For this review, take the finished solid that the model builds, in its own axes (mm). Face numbers are marked on the shaded views. Round coordinates to 2 decimals unless told otherwise and drop trailing zeros. Order: outer loops, then holes, each group sorted by start corner. A loop starts at its lowest first (then second) coordinate and runs counter-clockwise, first axis right, second up. Notation, with made-up numbers: (29.25, 32.25) -> (46.25, 32.25) arc R12 ccw to (46.25, 54.25) -> close; hole circle Ø6 at (-39, -12). An arc over 180 degrees is marked (long way). Answer in a Markdown table with one row per item.
```python
from build123d import *

# Parameters (mm, degrees)
SKETCH1_W           = 22
SKETCH1_H           = 6.5
SKETCH1_R           = 1.5
BOSS_EXTRUDE1_DEPTH = 2.5
FILLET4_R           = 2


with BuildPart() as part:
    # Sketch1 → Boss-Extrude1 (new body)
    with BuildSketch(Plane.XY):
        Rectangle(SKETCH1_W, SKETCH1_H)
        with Locations((-8.75, 0)):
            Circle(SKETCH1_R, mode=Mode.SUBTRACT)
        with Locations(Location((8.75, 0, 0), (0, 0, 180))):
            Circle(SKETCH1_R, mode=Mode.SUBTRACT)
    extrude(amount=BOSS_EXTRUDE1_DEPTH)

    # Fillet4
    fillet4_edges = [part.edges().sort_by_distance(p)[0] for p in [
        (11, -3.25, 1.25),
        (-11, -3.25, 1.25),
        (-11, 3.25, 1.25),
        (11, 3.25, 1.25),
    ]]
    fillet(fillet4_edges, radius=FILLET4_R)


solid = part.part
```
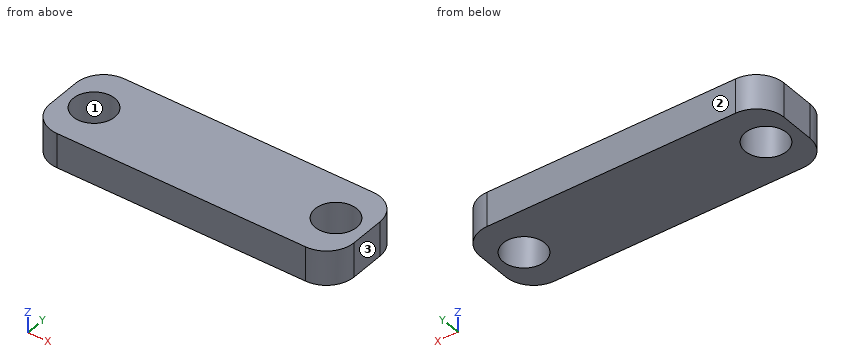
Q1. Take a section at D-D, the plane y = 0.25. Write out the cut boundary in (x, z).
Answer key:
| item | result |
|---|---|
| outline | (-11, 0) -> (-10.23, 0) -> (-10.23, 2.5) -> (-11, 2.5) -> close; (-7.27, 0) -> (7.27, 0) -> (7.27, 2.5) -> (-7.27, 2.5) -> close; (10.23, 0) -> (11, 0) -> (11, 2.5) -> (10.23, 2.5) -> close |
Q2. Take a section at A-A, the plane z = 0.6. Write out the cut boundary in (x, y), then the cut area to 3 significant figures.
Answer key:
| item | result |
|---|---|
| outline | (-11, -1.25) arc R2 ccw to (-9, -3.25) -> (9, -3.25) arc R2 ccw to (11, -1.25) -> (11, 1.25) arc R2 ccw to (9, 3.25) -> (-9, 3.25) arc R2 ccw to (-11, 1.25) -> close; hole circle Ø3 at (-8.75, 0); hole circle Ø3 at (8.75, 0) |
| area | 125 mm^2 |
Q3. The part is to be moulded in two halves that separate along X. For the marked faces 1, 2 and 3, say which applies: +X half, -X half, draft (parallel to the pull), parting line (faces both ways), or undercut.
Answer key:
| item | result |
|---|---|
| face 1 | undercut |
| face 2 | draft |
| face 3 | +X half |
Q4. Take a section at B-B, the plane x = 8.75. Write out the cut boundary in (y, z), then the cut area to 3 significant figures.
Answer key:
| item | result |
|---|---|
| outline | (-3.25, 0) -> (-1.5, 0) -> (-1.5, 2.5) -> (-3.25, 2.5) -> close; (1.5, 0) -> (3.25, 0) -> (3.25, 2.5) -> (1.5, 2.5) -> close |
| area | 8.75 mm^2 |
Q5. Take a section at C-C, the plane y = -0.75. Write out the cut boundary in (x, z), then the cut area to 3 significant figures.
Answer key:
| item | result |
|---|---|
| outline | (-11, 0) -> (-10.05, 0) -> (-10.05, 2.5) -> (-11, 2.5) -> close; (-7.45, 0) -> (7.45, 0) -> (7.45, 2.5) -> (-7.45, 2.5) -> close; (10.05, 0) -> (11, 0) -> (11, 2.5) -> (10.05, 2.5) -> close |
| area | 42.0 mm^2 |
Q6. To check wall thickness, follow probe 1 along Y at (x, z) = (-8.75, 1.2); probe 2 along X at (y, z) = (0.75, 0.3); probe 3 along X at (y, z) = (-0.25, 0.25). State the ranges of each line that lie inside material, in increasing order.
Answer key:
| item | result |
|---|---|
| probe 1 | y = -3.25 to -1.5, 1.5 to 3.25 |
| probe 2 | x = -11 to -10.05, -7.45 to 7.45, 10.05 to 11 |
| probe 3 | x = -11 to -10.23, -7.27 to 7.27, 10.23 to 11 |
Q7. Clearance check with a flat-ended pin moving along its axis: pin 1 Ø2.5 at (x, y) = (-8.75, 0) entering from +Z. State where the tip first meets the part, or that it passes through.
Answer key:
| item | result |
|---|---|
| pin 1 | passes through |
